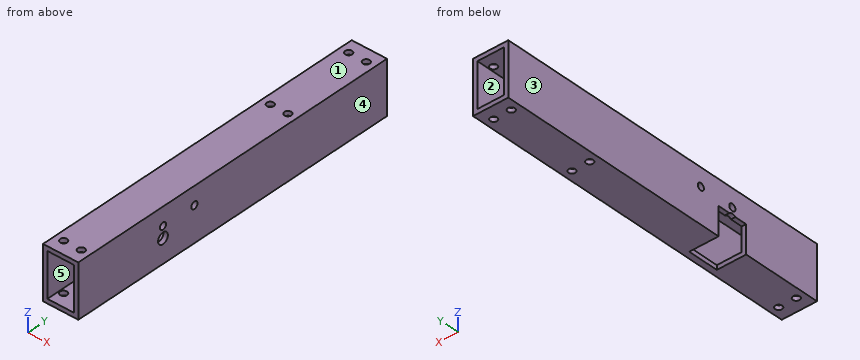
from build123d import *

# Parameters (mm, degrees)
SKETCH1_W           = 25.4
SKETCH1_H           = 38.1
SKETCH1_W_2         = 19.05
SKETCH1_H_2         = 31.75
EXTRUDE_THIN1_DEPTH = 248.92
SKETCH5_W           = 47.1424
SKETCH5_H           = 22.225
CUT_EXTRUDE2_DEPTH  = 21.082
SKETCH7_R           = 2.4892
CUT_EXTRUDE4_DEPTH  = 26.4
SKETCH8_R           = 2.4892
CUT_EXTRUDE5_DEPTH  = 26.4
SKETCH10_R          = 3.9624
CUT_EXTRUDE7_DEPTH  = 3.175
SKETCH11_R          = 3.9624
CUT_EXTRUDE8_DEPTH  = 77.2
SKETCH13_R          = 2.4892
CUT_EXTRUDE9_DEPTH  = 39.1
SKETCH16_R          = 2.4892
CUT_EXTRUDE13_DEPTH = 39.1


with BuildPart() as part:
    # Sketch1 → Extrude-Thin1 (new body)
    with BuildSketch(Plane(origin=(0, 0, 0), x_dir=(1, 0, 0), z_dir=(0, 1, 0))):
        with Locations((12.7, 19.05)):
            Rectangle(SKETCH1_W, SKETCH1_H)
        with Locations((12.7, 19.05)):
            Rectangle(SKETCH1_W_2, SKETCH1_H_2, mode=Mode.SUBTRACT)
    extrude(amount=EXTRUDE_THIN1_DEPTH)

    # Sketch5 → Cut-Extrude2 (cut)
    with BuildSketch(Plane.ZY):
        with Locations((-41.518281917, 68.2625)):
            Rectangle(SKETCH5_W, SKETCH5_H)
    extrude(amount=-CUT_EXTRUDE2_DEPTH, mode=Mode.SUBTRACT)

    # Sketch7 → Cut-Extrude4 (cut, through all)
    with BuildSketch(Plane.ZY):
        with Locations((-12.9032, 93.6625)):
            Circle(SKETCH7_R)
    extrude(amount=-CUT_EXTRUDE4_DEPTH, mode=Mode.SUBTRACT)

    # Sketch8 → Cut-Extrude5 (cut, through all)
    with BuildSketch(Plane.ZY):
        with Locations((-12.9032, 68.2625)):
            Circle(SKETCH8_R)
    extrude(amount=-CUT_EXTRUDE5_DEPTH, mode=Mode.SUBTRACT)

    # Sketch10 → Cut-Extrude7 (cut)
    with BuildSketch(Plane(origin=(25.4, 0, 0), x_dir=(0, 0, -1), z_dir=(1, 0, 0))):
        with Locations((21.0566, 68.2625)):
            Circle(SKETCH10_R)
    extrude(amount=-CUT_EXTRUDE7_DEPTH, mode=Mode.SUBTRACT)

    # Sketch11 → Cut-Extrude8 (cut, through all)
    with BuildSketch(Plane(origin=(76.2, 0, 0), x_dir=(0, 0, -1), z_dir=(1, 0, 0))):
        with Locations((21.0566, 68.2625)):
            Circle(SKETCH11_R)
    extrude(amount=-CUT_EXTRUDE8_DEPTH, mode=Mode.SUBTRACT)

    # Sketch13 → Cut-Extrude9 (cut, through all)
    with BuildSketch(Plane(origin=(0, 0, -38.1), x_dir=(-1, 0, 0), z_dir=(0, 0, -1))):
        with Locations((-19.05, 9.525)):
            Circle(SKETCH13_R)
        with Locations((-6.35, 9.525)):
            Circle(SKETCH13_R)
        with Locations((-6.35, 239.395)):
            Circle(SKETCH13_R)
        with Locations((-19.05, 239.395)):
            Circle(SKETCH13_R)
    extrude(amount=-CUT_EXTRUDE9_DEPTH, mode=Mode.SUBTRACT)

    # Sketch16 → Cut-Extrude13 (cut, through all)
    with BuildSketch(Plane(origin=(0, 0, -38.1), x_dir=(-1, 0, 0), z_dir=(0, 0, -1))):
        with Locations((-19.05, 176.15465)):
            Circle(SKETCH16_R)
        with Locations((-6.35, 176.15465)):
            Circle(SKETCH16_R)
    extrude(amount=-CUT_EXTRUDE13_DEPTH, mode=Mode.SUBTRACT)


solid = part.part
Verification items for the finished model (mm, model axes). Face numbers are marked on the shaded views. A direction names the side the tool comes from. Round coordinates to 2 decimals unless told otherwise and drop trailing zeros. Loops run counter-clockwise (first coordinate to the right, second up) from the corner with the lowest first, then second, coordinate; pieces in that order, holes last. Notation, with made-up numbers: (1.5, 41.25) - (52.5, 41.25) arc R27 cw to (52.5, 80.25) - close; hole circle Ø3 at (64, -26). An arc over 180 degrees is marked (long way). Use a Markdown table: item, result. Add a question column.
1. Access from +Z, -Z, +X, -X, +Y, -Y to the whole of each face (thin tool, end or side, straight path). Record for the marked faces 1 and 2.
2. Section check A-A, the plane y = 111. Record the boundary of the cut face in (x, z) (3 decimals), plus the area to 3 significant figures.
3. Thickness scan on probe 1 along Y at (x, z) = (6.35, -1.5); probe 2 along X at (y, z) = (101, -16) (3 decimals); probe 3 along Z at (x, y) = (9.5, 103) (3 decimals). Record the ranges inside material, lowest first. Write a range as [from, to].
4. Release check for a two-part mould opening along X. For the marked faces 3, 4 and 5 record: released by +X, released by -X, zero draft, split by the parting line, or undercut.
5. Section check B-B, the plane x = 6.35. Give the number of separate pieces and of enclosed holes in the cut face, plus the area to 3 significant figures.
6. Gauge pin test, flat ends, axial feed: pin 1 (2.5 mm diameter, centred on x = 2, y = 74, fed in from -Z); pin 2 (1 mm diameter, centred on y = 67.5, z = -37, fed in from -X). Record the tip position at first contact, or that the pin passes through.
Checks:
| question | item | result |
|---|---|---|
| 1 | face 1 | +Z, +X, -X, +Y, -Y |
| 1 | face 2 | +Y, -Y |
| 2 | outline | (0, -38.1) - (25.4, -38.1) - (25.4, 0) - (0, 0) - close; hole (3.175, -34.925) - (22.225, -34.925) - (22.225, -3.175) - (3.175, -3.175) - close |
| 2 | area | 363 mm^2 |
| 3 | probe 1 | y = [0, 7.04], [12.01, 173.67], [178.64, 236.91], [241.88, 248.92] |
| 3 | probe 2 | x = [0, 3.175], [22.225, 25.4] |
| 3 | probe 3 | z = [-38.1, -34.925], [-3.175, 0] |
| 4 | face 3 | released by -X |
| 4 | face 4 | released by +X |
| 4 | face 5 | undercut |
| 5 | separate pieces | 9 |
| 5 | enclosed holes | 0 |
| 5 | area | 1,420 mm^2 |
| 6 | pin 1 | stops at z = -17.95 |
| 6 | pin 2 | stops at x = 21.08 |
